The drawing under review shows one solid part. Ordinate dimensions are in mm from its lowest x, y, z. A direction names the side the tool comes from. Round coordinates to 2 decimals unless told otherwise and drop trailing zeros. Order: outer loops, then holes, each group sorted by start corner. A loop starts at its lowest first (then second) coordinate and runs counter-clockwise, first axis right, second up. Notation, with made-up numbers: M -26.5,11.5 L -0.5,11.5 A28 ccw -0.5,36.5 Z; hole C 31,64 d11. An arc over 180 degrees is marked long. Answer as a JSON object with one key per item and string values. Group by question number.
1) Insertion check: pin 1 Ø3 at (x, y) = (39, 13) entering from +Z; pin 2 Ø5 at (y, z) = (11.5, 130) entering from +X; pin 3 Ø10 at (x, y) = (189.5, 62) entering from +Z. Each pin has a flat end and moves straight along its axis. Give the tip position at first contact, or say it passes through.
2) Consider section D-D, the plane z = 139. Write out the cut boundary in (x, y).
3) Consider section A-A, the plane x = 50.8. Write out the cut boundary in (y, z), then the cut area to 3 significant figures.
4) The part is to be moulded in two halves that separate along X. For the marked faces 1, 2 and 3, say which applies: +X half, -X half, draft (parallel to the pull), parting line (faces both ways), or undercut.
5) Consider section B-B, the plane y = 44. Write out the cut boundary in (x, z), then the cut area to 3 significant figures.
6) To check wall thickness, follow line 1 (Z direction, x = 50.8, y = 42.5); line 2 (Y direction, x = 186.5, z = 29.5); line 3 (X direction, y = 93, z = 109). State the ranges of each line that lie inside material, in increasing order.
7) For the marked faces 4, 5 and 6, list the 3-axis set-ups (+Z, -Z, +X, -X, +Y, -Y) from which the entire face can be reached by the end or side of a thin tool; tool diameter is ignored.
8) Consider section C-C, the plane z = 20. Write out the cut boundary in (x, y).
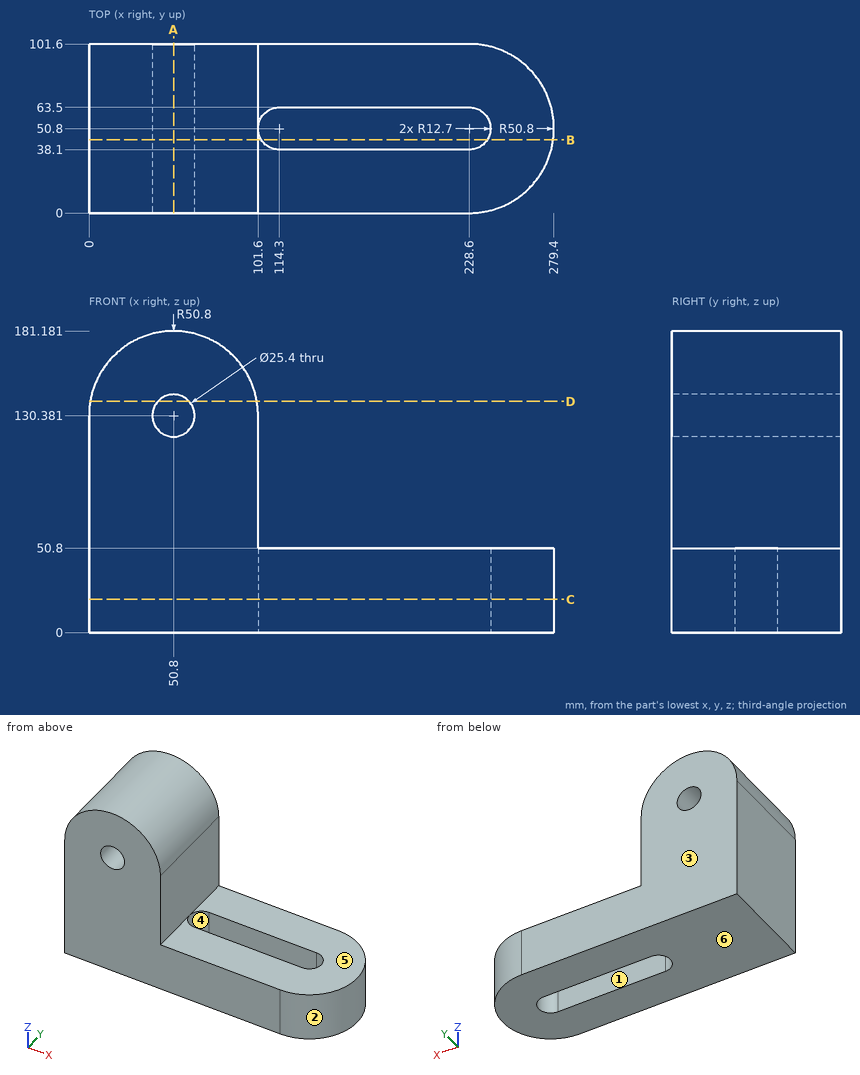
Results list:
{
 "1": {"pin 1": "z = 180.13", "pin 2": "x = 101.6", "pin 3": "z = 50.8"},
 "2": {"outline": "M 0.74,0 L 41.47,0 L 41.47,101.6 L 0.74,101.6 Z; M 60.13,0 L 100.86,0 L 100.86,101.6 L 60.13,101.6 Z"},
 "3": {"outline": "M 0,0 L 101.6,0 L 101.6,117.68 L 0,117.68 Z; M 0,143.08 L 101.6,143.08 L 101.6,181.18 L 0,181.18 Z", "area": "15,800 mm^2"},
 "4": {"face 1": "undercut", "face 2": "+X half", "face 3": "draft"},
 "5": {"outline": "M 0,0 L 103.57,0 L 103.57,50.8 L 101.6,50.8 L 101.6,130.38 A50.8 ccw 0,130.38 Z; M 239.33,0 L 278.94,0 L 278.94,50.8 L 239.33,50.8 Z; hole C 50.8,130.38 d25.4", "area": "18,900 mm^2"},
 "6": {"line 1": "0 to 117.68, 143.08 to 181.18", "line 2": "0 to 38.1, 63.5 to 101.6", "line 3": "0 to 101.6"},
 "7": {"face 4": "+Z, -Z", "face 5": "+Z, +X, +Y, -Y", "face 6": "-Z, +X, -X, +Y, -Y"},
 "8": {"outline": "M 0,0 L 228.6,0 A50.8 ccw 228.6,101.6 L 0,101.6 Z; hole M 114.3,38.1 L 228.6,38.1 A12.7 ccw 228.6,63.5 L 114.3,63.5 A12.7 ccw Z"}
}
